CAD build for the part. Positions are in the model's coordinates, mm. Coordinates: 2 decimals unless noted, no trailing zeros. Loops run counter-clockwise (first coordinate to the right, second up) from the corner with the lowest first, then second, coordinate; pieces in that order, holes last. Notation, with made-up numbers: (-26, -17.5) -> (-5, -17.5) arc R22 ccw to (-5, 10.5) -> close; hole circle Ø2 at (74, 61.5). An arc over 180 degrees is marked (long way). Answer as a JSON object with one key per item and string values. Group by question number.
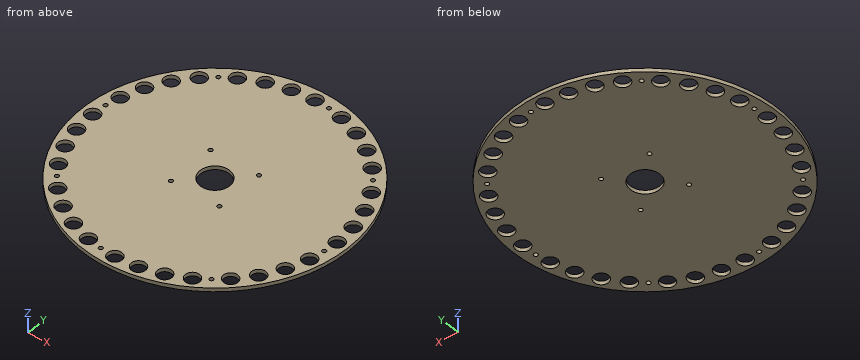
from build123d import *

# Parameters (mm, degrees)
F0_R            = 114.3
F0_R_2          = 1.7272
F0_R_3          = 12.7
F1_DEPTH        = 3.175
F2_R            = 6.1483621
F2_R_2          = 1.7272
F3_DEPTH        = 3.175
F3_COPIES_COUNT = 8


# Not quite as in the source:
# - a pattern or mirror of a feature is missing from the dataset's text; its kind, count and spacing are read off the source's solid


with BuildPart() as f1:
    # F0 (on Top) → F1 (new body)
    with BuildSketch(Plane.XY):
        Circle(F0_R)
        with Locations((-20.76684228, -20.76684228)):
            Circle(F0_R_2, mode=Mode.SUBTRACT)
        with Locations((20.76684228, -20.76684228)):
            Circle(F0_R_2, mode=Mode.SUBTRACT)
        with Locations((-20.76684228, 20.76684228)):
            Circle(F0_R_2, mode=Mode.SUBTRACT)
        Circle(F0_R_3, mode=Mode.SUBTRACT)
        with Locations((20.76684228, 20.76684228)):
            Circle(F0_R_2, mode=Mode.SUBTRACT)
    extrude(amount=F1_DEPTH)

    # F2 (on face) → F3 (cut, through all)
    with BuildSketch(Plane.XY.offset(3.175)):
        with Locations((-104.9766379, 0)):
            Circle(F2_R)
        with Locations((-103.2599191691, -18.9072366561)):
            Circle(F2_R)
        with Locations((-98.1659111494, -37.1960803446)):
            Circle(F2_R)
        with Locations((-89.8612219386, -54.2683636799)):
            Circle(F2_R)
        with Locations((-104.2084193553, 12.676744072)):
            Circle(F2_R_2)
    f3 = extrude(amount=-F3_DEPTH, mode=Mode.SUBTRACT)

    # F3_copies: F3 ×8 about axis
    f3_copies_axis = Axis((0, 0, 0), (0, 0, 1))
    for i in range(1, F3_COPIES_COUNT):
        add(f3.rotate(f3_copies_axis, i * 360 / F3_COPIES_COUNT), mode=Mode.SUBTRACT)


solid = f1.part
Item 1: Flat gauge pins, fed straight in: P1, Ø7.5, axis at x = 0, y = -104.98, coming from the +Z side; P2, Ø1, axis at y = 5.5, z = 2.5, coming from the -X side. Where does each tip first touch, or does it go through?
Item 2: Band-saw the part on C-C, the plane z = 2.65. Count the separate pieces of the cut face and the enclosed holes in it, and give its area (3 significant figures).
Item 3: Band-saw the part on A-A, the plane y = 0. List the corners of the cut face in (x, z) (3 decimals).
Item 4: Drill centre lines: L1, parallel to Y at x = -24, z = 2.8; L2, parallel to Y at x = 2, z = 0.9; L3, parallel to Y at x = -64.5, z = 1.4. Where is each one in solid material? Low to high.
Reply:
{
 "1": {"P1": "through", "P2": "x = -114.19"},
 "2": {"separate pieces": "1", "enclosed holes": "45", "area": "36,600 mm²"},
 "3": {"outline": "(-114.3, 0) -> (-111.125, 0) -> (-111.125, 3.175) -> (-114.3, 3.175) -> close; (-98.828, 0) -> (-12.7, 0) -> (-12.7, 3.175) -> (-98.828, 3.175) -> close; (12.7, 0) -> (98.828, 0) -> (98.828, 3.175) -> (12.7, 3.175) -> close; (111.125, 0) -> (114.3, 0) -> (114.3, 3.175) -> (111.125, 3.175) -> close"},
 "4": {"L1": "-111.75 to -107.95, -95.88 to 99.82, 106.7 to 111.75", "L2": "-114.28 to -110.79, -99.16 to -12.54, 12.54 to 99.16, 110.79 to 114.28", "L3": "-94.36 to -90.16, -82.61 to 80.94, 84.36 to 94.36"}
}
